```python
from build123d import *

# Parameters (mm, degrees)
EXTRUDE_START       = -20
EXTRUDE_1_OUTLINE_R = 10.5
EXTRUDE_1_DEPTH     = 20


# Read off the part's stored shape, not the designer's step: 填料-伸長1
with BuildPart() as part:
    # 填料-伸長1 outline → 填料-伸長1 (new body)
    with BuildSketch(Plane(origin=(26.04788271, 0, 0), x_dir=(0, 0, -1), z_dir=(1, 0, 0)).offset(EXTRUDE_START)):
        with BuildLine():
            Line((-201.999999965, -2.843045968), (-192.999999965, -2.843045968))
            Line((-192.999999965, -2.843045968), (-192.999999965, -22.843045968))
            ThreePointArc((-192.999999965, -22.843045968), (-179.999999965, -35.843045968), (-166.999999965, -22.843045968))
            Line((-166.999999965, -22.843045968), (-166.999999965, -2.843045968))
            Line((-166.999999965, -2.843045968), (-157.999999965, -2.843045968))
            Line((-157.999999965, -2.843045968), (-157.999999965, 2.156954032))
            Line((-157.999999965, 2.156954032), (-201.999999965, 2.156954032))
            Line((-201.999999965, 2.156954032), (-201.999999965, -2.843045968))
        make_face()
        with Locations((-179.999999965, -22.843045968)):
            Circle(EXTRUDE_1_OUTLINE_R, mode=Mode.SUBTRACT)
    extrude(amount=EXTRUDE_1_DEPTH)


solid = part.part
```
The model under review builds one solid part; all positions refer to its coordinate system, in mm. A direction names the side the tool comes from. Coordinates: 2 decimals unless noted, no trailing zeros. Order: outer loops, then holes, each group sorted by start corner. A loop starts at its lowest first (then second) coordinate and runs counter-clockwise, first axis right, second up. Notation, with made-up numbers: (-31, 0) -> (-13, 0) arc R17 ccw to (-13, 4) -> close; hole circle Ø9 at (50.5, 37). An arc over 180 degrees is marked (long way). Answer in a Markdown table with one row per item. Add a question column.
Item 1: Clearance check with flat-ended pins moving along their axes: pin 1 (1 mm diameter, centred on x = 20, z = 178.5, fed in from -Y); pin 2 (17 mm diameter, centred on y = -22.84, z = 180, fed in from -X); pin 3 (1.5 mm diameter, centred on x = 11.5, z = 165.5, fed in from -Y); pin 4 (10 mm diameter, centred on x = 17, z = 164, fed in from -Y). State where each tip first meets the part, or that it passes through.
Item 2: We need section D-D on z = 166. Write out the cut boundary in (x, y).
Item 3: We need section A-A on z = 180. Write out the cut boundary in (x, y), plus the area to 3 significant figures.
Item 4: Mouldability with a two-part tool opening along Z and no side actions: class faces 4 (the flat face through (16, 0, 158)), 5 (the flat face through (16, 2.157, 180)), 6 (the cylindrical face through (15.908, -19.689, 169.985)) as +Z half, -Z half, draft (parallel to the pull), parting line (faces both ways), or undercut.
Item 5: We need section B-B on x = 8.5. Write out the cut boundary in (y, z), plus the area to 3 significant figures.
Item 6: Machinability: for faces 1 (the flat face through (16, 0, 202)), 2 (the flat face through (16, -2.843, 163)), 3 (the flat face through (16, -13, 193)), which of the approach directions +Z, -Z, +X, -X, +Y, -Y give a long, thin tool a straight path to every point of the face, cutting with its end or side? Answer none if there is none.
Item 7: To check wall thickness, follow probe 1 along Y at (x, z) = (14.75, 179.5); probe 2 along Y at (x, z) = (21.25, 180); probe 3 along Z at (x, y) = (7, -7). State the ranges of each line that lie inside material, in increasing order.
Item 8: We need section C-C on y = -16.5. Write out the cut boundary in (x, z), plus the area to 3 significant figures.
Final values:
| question | item | result |
|---|---|---|
| 1 | pin 1 | stops at y = -35.8 |
| 1 | pin 2 | passes through |
| 1 | pin 3 | stops at y = -2.84 |
| 1 | pin 4 | stops at y = -29.77 |
| 2 | outline | (6.05, -2.84) -> (26.05, -2.84) -> (26.05, 2.16) -> (6.05, 2.16) -> close |
| 3 | outline | (6.05, -35.84) -> (26.05, -35.84) -> (26.05, -33.34) -> (6.05, -33.34) -> close; (6.05, -12.34) -> (26.05, -12.34) -> (26.05, 2.16) -> (6.05, 2.16) -> close |
| 3 | area | 340 mm2 |
| 4 | face 4 | -Z half |
| 4 | face 5 | draft |
| 4 | face 6 | undercut |
| 5 | outline | (-22.84, 167) -> (-2.84, 167) -> (-2.84, 158) -> (2.16, 158) -> (2.16, 202) -> (-2.84, 202) -> (-2.84, 193) -> (-22.84, 193) arc R13 ccw to start; hole circle Ø21 at (-22.84, 180) |
| 5 | area | 659 mm2 |
| 6 | face 1 | +Z, +X, -X, +Y, -Y |
| 6 | face 2 | -Z, +X, -X, -Y |
| 6 | face 3 | +Z, +X, -X, -Y |
| 7 | probe 1 | y = -35.83 to -33.33, -12.35 to 2.16 |
| 7 | probe 2 | y = -35.84 to -33.34, -12.34 to 2.16 |
| 7 | probe 3 | z = 167 to 193 |
| 8 | outline | (6.05, 167) -> (26.05, 167) -> (26.05, 171.63) -> (6.05, 171.63) -> close; (6.05, 188.37) -> (26.05, 188.37) -> (26.05, 193) -> (6.05, 193) -> close |
| 8 | area | 185 mm2 |
